Here's how the part is built. I have some questions about the finished solid (model axes, mm). Face numbers are marked on the shaded views. A direction names the side the tool comes from. Coordinates: 2 decimals unless noted, no trailing zeros. Loops run counter-clockwise (first coordinate to the right, second up) from the corner with the lowest first, then second, coordinate; pieces in that order, holes last. Notation, with made-up numbers: M 85,-0.75 L 111,-0.75 A17 cw 111,11.25 Z; hole C 25,3.5 d6. An arc over 180 degrees is marked long. Use one line per item in the form item = value. Start each with the question number.
(1) Imagine slicing it at D-D, the plane z = -9. Please give me the cut outline in (x, y).
(2) On a 3-axis mill with a long thin cutter (end or side, diameter ignored), from which of +Z, -Z, +X, -X, +Y, -Y can I reach the whole of each face in a straight line? I mean the marked faces 1, 2 and 3. Say none if no direction works.
(3) Imagine slicing it at A-A, the plane x = 0. Please give me the cut outline in (y, z).
(4) Will these pins go through, and if not, where does the flat tip stop? P1, Ø12, axis at y = 28.5, z = 7.5, coming from the -X side; P2, Ø20.5, axis at y = 11, z = -3, coming from the +X side; P3, Ø6, axis at x = 26, z = -13, coming from the -Y side; P4, Ø19.5, axis at x = -14, y = 11.5, coming from the +Z side.
(5) Imagine slicing it at C-C, the plane x = -29. Please give me the cut outline in (y, z).
(6) Imagine slicing it at B-B, the plane y = -12.5. Please give me the cut outline in (x, z), and give its area (3 significant figures).
(7) Please list where these lines run through material, in increasing order: L1, parallel to Y at x = 0, z = -9.5; L2, parallel to Y at x = -22, z = -14; L3, parallel to Z at x = 12, y = 45.5.
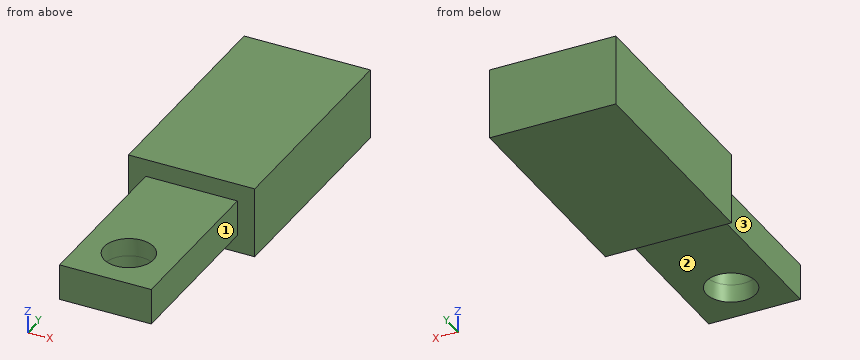
```python
from build123d import *

# Parameters (mm, degrees)
SKETCH1_W               = 64.516
SKETCH1_H               = 25.4
EXTRUDE2_DEPTH          = 59.309
EXTRUDE2_DEPTH_BACK     = 59.309
SKETCH2_R               = 17.399
CUT_EXTRUDE1_DEPTH      = 13.7
CUT_EXTRUDE1_DEPTH_BACK = 13.7
SKETCH3_W               = 88.9
SKETCH3_H               = 50.038
EXTRUDE3_DEPTH          = 159.258


with BuildPart() as part:
    # Sketch1 → Extrude2 (new body, two sides)
    with BuildSketch(Plane(origin=(0, 0, 0), x_dir=(1, 0, 0), z_dir=(0, 1, 0))) as extrude2_sk:
        Rectangle(SKETCH1_W, SKETCH1_H)
    extrude(amount=EXTRUDE2_DEPTH)
    extrude(extrude2_sk.sketch, amount=-EXTRUDE2_DEPTH_BACK)

    # Sketch2 → Cut-Extrude1 (cut, two sides)
    with BuildSketch(Plane.XY) as cut_extrude1_sk:
        with Locations((0, -27.051)):
            Circle(SKETCH2_R)
    extrude(amount=CUT_EXTRUDE1_DEPTH, mode=Mode.SUBTRACT)
    extrude(cut_extrude1_sk.sketch, amount=-CUT_EXTRUDE1_DEPTH_BACK, mode=Mode.SUBTRACT)

    # Sketch3 → Extrude3 (add)
    with BuildSketch(Plane(origin=(0, 59.309, 0), x_dir=(-1, 0, 0), z_dir=(0, 1, 0))):
        Rectangle(SKETCH3_W, SKETCH3_H)
    extrude(amount=EXTRUDE3_DEPTH)


solid = part.part
```
Answer:
q1.outline = M -44.45,59.31 L -32.26,59.31 L -32.26,-59.31 L 32.26,-59.31 L 32.26,59.31 L 44.45,59.31 L 44.45,218.57 L -44.45,218.57 Z; hole C 0,-27.05 d34.8
q2.face_1 = +Z, -Z, +X, -Y
q2.face_2 = -Z, +X, -X, -Y
q2.face_3 = +Z, -Z, -X, -Y
q3.outline = M -59.31,-12.7 L -44.45,-12.7 L -44.45,12.7 L -59.31,12.7 Z; M -9.65,-12.7 L 59.31,-12.7 L 59.31,-25.02 L 218.57,-25.02 L 218.57,25.02 L 59.31,25.02 L 59.31,12.7 L -9.65,12.7 Z
q4.P1 = -32.26
q4.P2 = 32.26
q4.P3 = -59.31
q4.P4 = 12.7
q5.outline = M -59.31,-12.7 L 59.31,-12.7 L 59.31,-25.02 L 218.57,-25.02 L 218.57,25.02 L 59.31,25.02 L 59.31,12.7 L -59.31,12.7 Z
q6.outline = M -32.26,-12.7 L -9.54,-12.7 L -9.54,12.7 L -32.26,12.7 Z; M 9.54,-12.7 L 32.26,-12.7 L 32.26,12.7 L 9.54,12.7 Z
q6.area = 1,150 mm²
q7.L1 = -59.31 to -44.45, -9.65 to 218.57
q7.L2 = 59.31 to 218.57
q7.L3 = -12.7 to 12.7
